Verification items for the finished model (mm, model axes). A direction names the side the tool comes from. Coordinates: 2 decimals unless noted, no trailing zeros. Loops run counter-clockwise (first coordinate to the right, second up) from the corner with the lowest first, then second, coordinate; pieces in that order, holes last. Notation, with made-up numbers: (50.25, -33) -> (78.25, -33) arc R7 cw to (78.25, -20) -> close; hole circle Ø8 at (-14.5, -40). An arc over 180 degrees is marked (long way). Answer as a JSON object with one key per item and string values. Group by question number.
Q1. Set-up check for faces 4 (the flat face through (0.389, 5.521, 2.483)), 5 (the flat face through (-2, 3, 0)): record each of +Z, -Z, +X, -X, +Y, -Y from which the full face is reachable in a straight line by a thin tool's end or side.
Q2. Cross-section at D-D on z = 5.75. Record the boundary of the cut face in (x, y) (3 decimals), and give its area (3 significant figures).
Q3. Cross-section at C-C on y = 5.5. Record the boundary of the cut face in (x, z).
Q4. Release check for a two-part mould opening along Z. For faces 1 (the cylindrical face through (-0.97, 6.58, 1.92)), 2 (the cylindrical face through (-0.69, -3.1, 3.13)), 3 (the flat face through (0, 4, 3)) record: released by +Z, released by -Z, zero draft, split by the parting line, or undercut.
Q5. Cross-section at B-B on x = -3. Record the boundary of the cut face in (y, z), and give its area (3 significant figures).
Q6. Gauge pin test, flat end, axial feed: pin 1 Ø3 at (x, z) = (-3.5, 3.5) entering from +Y. Record the tip position at first contact, or that the pin passes through.
Q7. Cross-section at A-A on y = 0. Record the boundary of the cut face in (x, z) (3 decimals).
Q8. Scan lines: L1, parallel to X at y = 5.5, z = 4.25; L2, parallel to Y at x = 0, z = 4 (3 decimals); L3, parallel to Y at x = -2.25, z = 2.5. Record each from-to range of solid material in increasing order.
```python
from build123d import *

# Parameters (mm, degrees)
SKETCH1_R            = 6.35
SKETCH1_R_2          = 3.175
BODY_DEPTH           = 6.35
SET_SCREW_REACH      = 18.089
SET_SCREW_END_RADIUS = 6.35
SKETCH2_R            = 1.5875
HEX_KEY_DEPTH        = 3


with BuildPart() as part:
    # Sketch1 → Body (new body)
    with BuildSketch(Plane.XY):
        Circle(SKETCH1_R)
        Circle(SKETCH1_R_2, mode=Mode.SUBTRACT)
    extrude(amount=BODY_DEPTH)

    # Set Screw: up to this cylinder (the profile starts outside it)
    set_screw_end = Plane(origin=(0, 0, 3.175), z_dir=(0, 0, -1)) * Cylinder(SET_SCREW_END_RADIUS, 49.878, mode=Mode.PRIVATE)
    # Sketch2 → Set Screw (add, up to the surface)
    with BuildSketch(Plane(origin=(0, 7, 0), x_dir=(1, 0, 0), z_dir=(0, 1, 0)), mode=Mode.PRIVATE) as set_screw_sk1:
        with Locations(Location((0, -3.175, 0), (0, 0, 270))):
            Circle(SKETCH2_R)
    set_screw_tool1 = extrude(set_screw_sk1.sketch, amount=-SET_SCREW_REACH, mode=Mode.PRIVATE) - set_screw_end
    add(set_screw_tool1.solids().sort_by_distance((0, 7, 3.175))[0])

    # Sketch3 → Hex Key (cut)
    with BuildSketch(Plane(origin=(0, 7, 0), x_dir=(1, 0, 0), z_dir=(0, 1, 0))):
        Polygon((0.802721832, -3.617368334), (0.784463132, -2.701006668), (-0.018258701, -2.258638334), (-0.802721832, -2.732631666), (-0.784463132, -3.648993332), (0.018258701, -4.091361666), align=None)
    extrude(amount=-HEX_KEY_DEPTH, mode=Mode.SUBTRACT)


solid = part.part
```
Computed values:
{
 "1": {"face 4": "+Y", "face 5": "-Z, +X, -X, +Y, -Y"},
 "2": {"outline": "circle Ø12.7 at (0, 0); hole circle Ø6.35 at (0, 0)", "area": "95.0 mm²"},
 "3": {"outline": "(-3.17, 0) -> (3.17, 0) -> (3.17, 6.35) -> (-3.17, 6.35) -> close; hole (-0.8, 2.73) -> (-0.02, 2.26) -> (0.78, 2.7) -> (0.8, 3.62) -> (0.02, 4.09) -> (-0.78, 3.65) -> close"},
 "4": {"face 1": "split by the parting line", "face 2": "zero draft", "face 3": "undercut"},
 "5": {"outline": "(-5.6, 0) -> (-1.04, 0) -> (-1.04, 6.35) -> (-5.6, 6.35) -> close; (1.04, 0) -> (5.6, 0) -> (5.6, 6.35) -> (1.04, 6.35) -> close", "area": "57.9 mm²"},
 "6": {"pin 1": "stops at y = 6.03"},
 "7": {"outline": "(-6.35, 0) -> (-3.175, 0) -> (-3.175, 6.35) -> (-6.35, 6.35) -> close; (3.175, 0) -> (6.35, 0) -> (6.35, 6.35) -> (3.175, 6.35) -> close"},
 "8": {"L1": "x = -3.17 to 3.17", "L2": "y = -6.35 to -3.175, 3.175 to 4", "L3": "y = -5.94 to -2.24, 2.24 to 5.94"}
}
